Geometry: final body of the model. Coordinates: model frame, mm. A direction names the side the tool comes from. Give positions to 0.01 mm unless a question says otherwise; leave off trailing zeros. One line per question, with ' | ' between items.
from build123d import *

# Parameters (mm, degrees)
SKETCH_1_W          = 1000
SKETCH_1_H          = 1000
EXTRUDE_1_DEPTH     = 50
SKETCH_2_W          = 50
SKETCH_2_H          = 50
CUT_EXTRUDE_1_DEPTH = 709.872343938
SKETCH_3_W          = 50
SKETCH_3_H          = 50
CUT_EXTRUDE_2_DEPTH = 709.872343938
SKETCH_4_W          = 50
SKETCH_4_H          = 50
CUT_EXTRUDE_3_DEPTH = 709.872343938
SKETCH_5_W          = 50
SKETCH_5_H          = 50
CUT_EXTRUDE_4_DEPTH = 709.872343938


with BuildPart() as part:
    # 草图1 → 凸台-拉伸1 (new body)
    with BuildSketch(Plane.XY):
        Rectangle(SKETCH_1_W, SKETCH_1_H)
    extrude(amount=EXTRUDE_1_DEPTH)

    # 草图2 → 切除-拉伸1 (cut, through all)
    with BuildSketch(Plane.XY):
        with Locations((450, 450)):
            Rectangle(SKETCH_2_W, SKETCH_2_H)
    extrude(amount=CUT_EXTRUDE_1_DEPTH, mode=Mode.SUBTRACT)

    # 草图3 → 切除-拉伸2 (cut, through all)
    with BuildSketch(Plane.XY):
        with Locations((-450, 450)):
            Rectangle(SKETCH_3_W, SKETCH_3_H)
    extrude(amount=CUT_EXTRUDE_2_DEPTH, mode=Mode.SUBTRACT)

    # 草图4 → 切除-拉伸3 (cut, through all)
    with BuildSketch(Plane.XY):
        with Locations((450, -450)):
            Rectangle(SKETCH_4_W, SKETCH_4_H)
    extrude(amount=CUT_EXTRUDE_3_DEPTH, mode=Mode.SUBTRACT)

    # 草图5 → 切除-拉伸4 (cut, through all)
    with BuildSketch(Plane.XY):
        with Locations((-450, -450)):
            Rectangle(SKETCH_5_W, SKETCH_5_H)
    extrude(amount=CUT_EXTRUDE_4_DEPTH, mode=Mode.SUBTRACT)


solid = part.part
(1) Set-up query: faces 5 (the face through (-7, 7, 50)), 6 (the face through (-475, 450, 25)). Return all of +Z, -Z, +X, -X, +Y, -Y with unobstructed straight access to the full face (end or side cutting, diameter ignored); none if empty.
Working result:
face 5: +Z, +X, -X, +Y, -Y | face 6: +Z, -Z
(2) Draft query along Y for faces 1 (the face through (-450, -475, 25)), 2 (the face through (-500, -7, 25)), 3 (the face through (-7, 500, 25)), 4 (the face through (-7, -500, 25)). Return one class per face: released by +Y, released by -Y, zero draft, split by the parting line, or undercut.
Working result:
face 1: undercut | face 2: zero draft | face 3: released by +Y | face 4: released by -Y
(3) Material intervals for L1, parallel to Y at x = -437, z = 30, sorted ascending. Write a range as [from, to].
Working result:
L1: y = [-500, -475], [-425, 425], [475, 500]
